Source: CAD feature listing. Evaluate the final solid. Frame: model axes, mm. A direction names the side the tool comes from. Coordinates: 2 decimals unless noted, no trailing zeros. Order: outer loops, then holes, each group sorted by start corner. A loop starts at its lowest first (then second) coordinate and runs counter-clockwise, first axis right, second up. Notation, with made-up numbers: (74, -33) -> (102, -33) arc R8 cw to (102, -22) -> close; hole circle Ø4 at (-30, 3). An arc over 180 degrees is marked (long way). Write each question's results on one line, items separated by ' | '. Start each with the question number.
from build123d import *

# Parameters (mm, degrees)
SKETCH1_W           = 55
SKETCH1_H           = 55
SKETCH1_R           = 4.75
SKETCH1_R_2         = 2.15
BOSS_EXTRUDE1_DEPTH = 19.5
CUT_EXTRUDE10_DEPTH = 3.5
SKETCH5_R           = 15.392304845
CUT_EXTRUDE2_DEPTH  = 18
SKETCH6_OUTSIDE_W   = 73.038
SKETCH6_OUTSIDE_H   = 73.038
CUT_EXTRUDE3_DEPTH  = 10.5
SKETCH7_R           = 1.75
CUT_EXTRUDE4_DEPTH  = 9
CUT_EXTRUDE6_REACH  = 73.751
CUT_EXTRUDE11_REACH = 86.299
FILLET2_R           = 2
FILLET3_R           = 1


with BuildPart() as part:
    # Sketch1 → Boss-Extrude1 (new body)
    with BuildSketch(Plane.XY):
        with Locations((27.5, 27.5)):
            Rectangle(SKETCH1_W, SKETCH1_H)
        with Locations((27.5, 27.5)):
            Circle(SKETCH1_R, mode=Mode.SUBTRACT)
        with Locations((8, 47)):
            Circle(SKETCH1_R_2, mode=Mode.SUBTRACT)
        with Locations((47, 47)):
            Circle(SKETCH1_R_2, mode=Mode.SUBTRACT)
        with Locations((41, 8)):
            Circle(SKETCH1_R_2, mode=Mode.SUBTRACT)
        with Locations((14, 8)):
            Circle(SKETCH1_R_2, mode=Mode.SUBTRACT)
    extrude(amount=BOSS_EXTRUDE1_DEPTH)

    # Sketch11 → Cut-Extrude10 (cut)
    with BuildSketch(Plane.XY):
        Polygon((10.049593456, 50.55), (5.950406544, 50.55), (3.900813089, 47), (5.950406544, 43.45), (10.049593456, 43.45), (12.099186911, 47), align=None)
        Polygon((42.900813089, 47), (44.950406544, 50.55), (49.049593456, 50.55), (51.099186911, 47), (49.049593456, 43.45), (44.950406544, 43.45), align=None)
        Polygon((38.950406544, 11.55), (43.049593456, 11.55), (45.099186911, 8), (43.049593456, 4.45), (38.950406544, 4.45), (36.900813089, 8), align=None)
        Polygon((11.950406544, 11.55), (16.049593456, 11.55), (18.099186911, 8), (16.049593456, 4.45), (11.950406544, 4.45), (9.900813089, 8), align=None)
    extrude(amount=CUT_EXTRUDE10_DEPTH, mode=Mode.SUBTRACT)

    # Sketch5 → Cut-Extrude2 (cut)
    with BuildSketch(Plane.XY.offset(19.5)):
        with Locations((27.5, 27.5)):
            Circle(SKETCH5_R)
    extrude(amount=-CUT_EXTRUDE2_DEPTH, mode=Mode.SUBTRACT)

    # Sketch6 outside → Cut-Extrude3 (cut)
    with BuildSketch(Plane.XY.offset(19.5)):
        with Locations((27.5, 27.5)):
            Rectangle(SKETCH6_OUTSIDE_W, SKETCH6_OUTSIDE_H)
        with BuildLine():
            Line((12.44308051, 19.732705171), (4.925539544, 22.468866318))
            Line((4.925539544, 22.468866318), (4.925539544, 27.468866318))
            Line((4.925539544, 27.468866318), (0, 27.468866318))
            Line((0, 27.468866318), (0, 10.397959841))
            Line((0, 10.397959841), (8.457233587, 7.319778551))
            Line((8.457233587, 7.319778551), (8.457233587, 0))
            Line((8.457233587, 0), (46.542766413, 0))
            Line((46.542766413, 0), (46.542766413, 7.319778551))
            Line((46.542766413, 7.319778551), (55, 10.397959841))
            Line((55, 10.397959841), (55, 27.468866318))
            Line((55, 27.468866318), (50.074460456, 27.468866318))
            Line((50.074460456, 27.468866318), (50.074460456, 22.468866318))
            Line((50.074460456, 22.468866318), (42.55691949, 19.732705171))
            ThreePointArc((42.55691949, 19.732705171), (27.5, 10.557695155), (12.44308051, 19.732705171))
        make_face(mode=Mode.SUBTRACT)
    extrude(amount=-CUT_EXTRUDE3_DEPTH, mode=Mode.SUBTRACT)

    # Sketch7 → Cut-Extrude4 (cut)
    with BuildSketch(Plane.XY):
        with Locations((10, 35.5)):
            Circle(SKETCH7_R)
        with Locations((45, 35.5)):
            Circle(SKETCH7_R)
    extrude(amount=CUT_EXTRUDE4_DEPTH, mode=Mode.SUBTRACT)

    # Sketch9 → Cut-Extrude6 (cut, up to next)
    with BuildSketch(Plane(origin=(3.341839876, 9.181629599, 0), x_dir=(0, 0, 1), z_dir=(-0.3420201433256653, -0.9396926207859098, 0)), mode=Mode.PRIVATE) as cut_extrude6_sk1:
        with BuildLine():
            Line((14.25, 2.056311715), (19.5, 2.056311715))
            Line((19.5, 2.056311715), (19.5, -0.943688285))
            Line((19.5, -0.943688285), (14.25, -0.943688285))
            ThreePointArc((14.25, -0.943688285), (12.75, 0.556311715), (14.25, 2.056311715))
        make_face()
    cut_extrude6_tool1 = extrude(cut_extrude6_sk1.sketch, amount=-CUT_EXTRUDE6_REACH, mode=Mode.PRIVATE) & part.part
    add(cut_extrude6_tool1.solids().sort_by_distance((2.819078, 9.371899, 16.277233))[0], mode=Mode.SUBTRACT)

    # Sketch10 → Cut-Extrude11 (cut, up to next)
    with BuildSketch(Plane(origin=(3.091937938, -8.495029668, 0), x_dir=(0, 0, -1), z_dir=(0.3420201433256654, -0.9396926207859098, 0)), mode=Mode.PRIVATE) as cut_extrude11_sk1:
        with BuildLine():
            Line((-14.25, 53.739405858), (-19.5, 53.739405858))
            Line((-19.5, 53.739405858), (-19.5, 50.739405858))
            Line((-19.5, 50.739405858), (-14.25, 50.739405858))
            ThreePointArc((-14.25, 50.739405858), (-12.75, 52.239405858), (-14.25, 53.739405858))
        make_face()
    cut_extrude11_tool1 = extrude(cut_extrude11_sk1.sketch, amount=-CUT_EXTRUDE11_REACH, mode=Mode.PRIVATE) & part.part
    add(cut_extrude11_tool1.solids().sort_by_distance((52.180922, 9.371899, 16.277233))[0], mode=Mode.SUBTRACT)

    # Fillet2
    fillet2_edges = [part.edges().sort_by_distance(p)[0] for p in [
        (0, 55, 4.5),
        (55, 55, 4.5),
        (55, 0, 4.5),
        (0, 0, 4.5),
        (27.5, 55, 0),
        (55, 27.5, 0),
        (27.5, 0, 0),
        (0, 27.5, 0),
    ]]
    fillet(fillet2_edges, radius=FILLET2_R)

    # Fillet3
    fillet3_edges = [part.edges().sort_by_distance(p)[0] for p in [
        (0, 10.397959841, 14.25),
        (12.44308051, 19.732705171, 14.25),
        (42.55691949, 19.732705171, 14.25),
        (55, 10.397959841, 14.25),
        (46.542766413, 7.319778551, 14.25),
        (46.542766413, 0, 14.25),
        (8.457233587, 0, 14.25),
        (8.457233587, 7.319778551, 14.25),
    ]]
    fillet(fillet3_edges, radius=FILLET3_R)


solid = part.part
(1) First-contact query: P1, Ø12, axis at x = 16, y = 23, coming from the -Z side; P2, Ø6, axis at y = 4, z = 15, coming from the -X side. Flat tips, straight axial feed; report the tip coordinate or a pass-through.
(2) Section A-A on x = 27.5. Return the cut outline in (y, z).
(3) Line query: L1, parallel to X at y = 34.5, z = 8.75; L2, parallel to Y at x = 8, z = 5.3; L3, parallel to Y at x = 45, z = 3.25. Output: solid intervals per line, ascending.
(4) Reachability of faces 1 (the cylindrical face through (32.03, 28.93, 0.74)), 2 (the flat face through (24, 24, 1.5)), 3 (the cylindrical face through (27.75, 10.56, 14.32)), 4 (the flat face through (8, 50.55, 2)) from +Z, -Z, +X, -X, +Y, -Y: full face, straight path, thin tool, end or side. Return the list, or none.
(5) Section C-C on z = 7.25. Return the cut outline in (x, y).
(6) Section B-B on y = 34.5. Return the cut outline in (x, z), then the cut area to 3 significant figures.
(7) Section D-D on z = 10.25. Return the cut outline in (x, y), then the cut area to 4 significant figures.
(8) Draft query along Y for faces 5 (the flat face through (41, 4.45, 2)), 6 (the flat face through (21, 43, 9)), 7 (the flat face through (51.4, 15.9, 16.8)), 8 (the cylindrical face through (27.86, 0.6, 0.57)). Return one class per face: released by +Y, released by -Y, zero draft, split by the parting line, or undercut.
Results list:
1) P1: stops at z = 0 | P2: stops at x = 8.38
2) outline: (0, 2) arc R2 ccw to (2, 0) -> (22.75, 0) -> (22.75, 1.5) -> (12.11, 1.5) -> (12.11, 9) -> (10.56, 9) -> (10.56, 19.5) -> (0, 19.5) -> close; (32.25, 0) -> (53, 0) arc R2 ccw to (55, 2) -> (55, 9) -> (42.89, 9) -> (42.89, 1.5) -> (32.25, 1.5) -> close
3) L1: x = 0 to 8.56, 11.44 to 13.79, 41.21 to 43.56, 46.44 to 55 | L2: y = 0 to 44.85, 49.15 to 55 | L3: y = 0 to 7.83, 8.17 to 33.75, 37.25 to 43.45, 50.55 to 55
4) face 1: +Z, -Z | face 2: +Z | face 3: +Z, +Y | face 4: -Z
5) outline: (0, 2) arc R2 ccw to (2, 0) -> (53, 0) arc R2 ccw to (55, 2) -> (55, 53) arc R2 ccw to (53, 55) -> (2, 55) arc R2 ccw to (0, 53) -> close; hole circle Ø4.3 at (8, 47); hole circle Ø3.5 at (10, 35.5); hole circle Ø4.3 at (14, 8); hole circle Ø30.78 at (27.5, 27.5); hole circle Ø4.3 at (41, 8); hole circle Ø3.5 at (45, 35.5); hole circle Ø4.3 at (47, 47)
6) outline: (0, 2) arc R2 ccw to (2, 0) -> (8.56, 0) -> (8.56, 9) -> (0, 9) -> close; (11.44, 0) -> (43.56, 0) -> (43.56, 9) -> (41.21, 9) -> (41.21, 1.5) -> (13.79, 1.5) -> (13.79, 9) -> (11.44, 9) -> close; (46.44, 0) -> (53, 0) arc R2 ccw to (55, 2) -> (55, 9) -> (46.44, 9) -> close | area: 236 mm²
7) outline: (0, 11.1) arc R1 ccw to (0.66, 10.16) -> (7.8, 7.56) arc R1 cw to (8.46, 6.62) -> (8.46, 1) arc R1 ccw to (9.46, 0) -> (45.54, 0) arc R1 ccw to (46.54, 1) -> (46.54, 6.62) arc R1 cw to (47.2, 7.56) -> (54.34, 10.16) arc R1 ccw to (55, 11.1) -> (55, 27.47) -> (50.07, 27.47) -> (50.07, 22.47) -> (42.92, 19.86) arc R1 ccw to (42.38, 19.4) arc R16.94 cw to (12.62, 19.4) arc R1 ccw to (12.08, 19.86) -> (4.93, 22.47) -> (4.93, 27.47) -> (0, 27.47) -> close; hole circle Ø4.3 at (14, 8); hole circle Ø4.3 at (41, 8) | area: 805.5 mm²
8) face 5: undercut | face 6: zero draft | face 7: undercut | face 8: released by -Y
